```python
from build123d import *

# Parameters (mm, degrees)
SKETCH1_R           = 1.5875
BOSS_EXTRUDE1_DEPTH = 5
SKETCH2_R           = 6
SKETCH2_R_2         = 3.175
BOSS_EXTRUDE2_DEPTH = 20
FILLET1_R           = 5
FILLET2_R           = 1
SKETCH3_R           = 1.5875
CUT_EXTRUDE1_DEPTH  = 16
FILLET3_R           = 1
SKETCH4_R           = 3.175
CUT_EXTRUDE2_DEPTH  = 6


with BuildPart() as part:
    # Sketch1 → Boss-Extrude1 (new body)
    with BuildSketch(Plane(origin=(0, 0, 0), x_dir=(0, 0, -1), z_dir=(1, 0, 0))):
        Polygon((-24.516144589, 8.853546087), (13.583855411, 8.853546087), (13.583855411, 23.853546087), (-24.516144589, 23.853546087), (-44.516144589, 23.853546087), (-44.516144589, 8.853546087), align=None)
        with Locations((-18.166144589, 16.353546087)):
            Circle(SKETCH1_R, mode=Mode.SUBTRACT)
        with Locations((7.233855411, 16.353546087)):
            Circle(SKETCH1_R, mode=Mode.SUBTRACT)
        with Locations((-38.166144589, 16.353546087)):
            Circle(SKETCH1_R, mode=Mode.SUBTRACT)
    extrude(amount=BOSS_EXTRUDE1_DEPTH)

    # Sketch2 → Boss-Extrude2 (add)
    with BuildSketch(Plane(origin=(5, 0, 0), x_dir=(0, 0, -1), z_dir=(1, 0, 0))):
        with Locations((-5.466144589, 16.353546087)):
            Circle(SKETCH2_R)
        with Locations((-5.466144589, 16.353546087)):
            Circle(SKETCH2_R_2, mode=Mode.SUBTRACT)
    extrude(amount=BOSS_EXTRUDE2_DEPTH)

    # Fillet1
    fillet1_edges = [part.edges().sort_by_distance(p)[0] for p in [
        (2.5, 8.853546087, 44.516144589),
        (2.5, 23.853546087, 44.516144589),
        (2.5, 23.853546087, -13.583855411),
        (2.5, 8.853546087, -13.583855411),
    ]]
    fillet(fillet1_edges, radius=FILLET1_R)

    # Fillet2
    fillet2_edges = [part.edges().sort_by_distance(p)[0] for p in [
        (25, 16.353546087, 11.466144589),
    ]]
    fillet(fillet2_edges, radius=FILLET2_R)

    # Sketch3 → Cut-Extrude1 (cut, through all)
    with BuildSketch(Plane(origin=(0, 23.853546087, 0), x_dir=(1, 0, 0), z_dir=(0, 1, 0))):
        with Locations((15, -5.466144589)):
            Circle(SKETCH3_R)
    extrude(amount=-CUT_EXTRUDE1_DEPTH, mode=Mode.SUBTRACT)

    # Fillet3
    fillet3_edges = [part.edges().sort_by_distance(p)[0] for p in [
        (5, 8.853546087, 15.466144589),
        (5, 16.353546087, 44.516144589),
        (5, 16.353546087, -13.583855411),
        (5, 23.853546087, 15.466144589),
        (5, 22.389079993, -12.119389316),
        (5, 10.318012181, -12.119389316),
        (5, 22.389079993, 43.051678495),
        (5, 10.318012181, 43.051678495),
    ]]
    fillet(fillet3_edges, radius=FILLET3_R)

    # Sketch4 → Cut-Extrude2 (cut, through all)
    with BuildSketch(Plane(origin=(5, 0, 0), x_dir=(0, 0, -1), z_dir=(1, 0, 0))):
        with Locations((-5.466144589, 16.353546087)):
            Circle(SKETCH4_R)
    extrude(amount=-CUT_EXTRUDE2_DEPTH, mode=Mode.SUBTRACT)


solid = part.part
```
The model under review builds one solid part; all positions refer to its coordinate system, in mm. Give positions to 0.01 mm unless a question says otherwise; leave off trailing zeros. Write each loop counter-clockwise with the first axis right and the second up, starting at its lowest first coordinate (ties: lowest second). Pieces come first, ordered by that corner, then holes. Notation, with made-up numbers: M -36,19 L -17,19 A12 cw -17,28 Z; hole C 87.25,26.5 d9. An arc over 180 degrees is marked long. Answer in a Markdown table with one row per item.
Item 1: Draft analysis for pull direction Z (two halves, no side actions). For faces 1 (the face through (0, 16, 16)), 2 (the face through (15.853, 20.754, 4.128)), 3 (the face through (2.028, 10.279, 43.013)), state which applies: +Z half, -Z half, draft (parallel to the pull), parting line (faces both ways), or undercut.
Check sheet entries:
| item | result |
|---|---|
| face 1 | draft |
| face 2 | undercut |
| face 3 | +Z half |
Item 2: Add section A-A on x = 15. Give the boundary of the cut face in (y, z) (3 decimals), plus the area to 3 significant figures.
Check sheet entries:
| item | result |
|---|---|
| outline | M 10.567,3.879 A6 ccw 22.14,3.879 L 19.103,3.879 A3.175 cw 13.604,3.879 Z; M 10.567,7.054 L 13.604,7.054 A3.175 cw 19.103,7.054 L 22.14,7.054 A6 ccw Z |
| area | 63.1 mm2 |
Item 3: For P1, Ø4, axis at x = 15, z = 5.47, coming from the +Y side; P2, Ø12, axis at x = 16.5, z = -2.5, coming from the -Y side; P3, Ø1.5, axis at y = 17, z = 14.5, coming from the +X side, all flat-tipped, find the tip position at first contact; note any pin that passes through.
Check sheet entries:
| item | result |
|---|---|
| P1 | y = 22.35 |
| P2 | y = 10.68 |
| P3 | x = 5 |
Item 4: Add section B-B on z = 37.5. Give the boundary of the cut face in (x, y).
Check sheet entries:
| item | result |
|---|---|
| outline | M 0,8.85 L 4,8.85 A1 ccw 5,9.85 L 5,14.91 L 0,14.91 Z; M 0,17.79 L 5,17.79 L 5,22.85 A1 ccw 4,23.85 L 0,23.85 Z |
Item 5: Add section C-C on y = 17.25. State how many separate pieces and enclosed holes the cut face has, plus the area to 3 significant figures.
Check sheet entries:
| item | result |
|---|---|
| separate pieces | 5 |
| enclosed holes | 0 |
| area | 335 mm2 |
Item 6: For line 1 along X through (y, z) = (15, -2); line 2 along Z through (x, y) = (15, 20.5); line 3 along Z through (x, y) = (21.5, 18.25), list the stretches that pass through material, from the lowest coordinate up.
Check sheet entries:
| item | result |
|---|---|
| line 1 | 0 to 5 |
| line 2 | 1.13 to 3.88, 7.05 to 9.8 |
| line 3 | -0.23 to 2.92, 8.01 to 11.16 |
